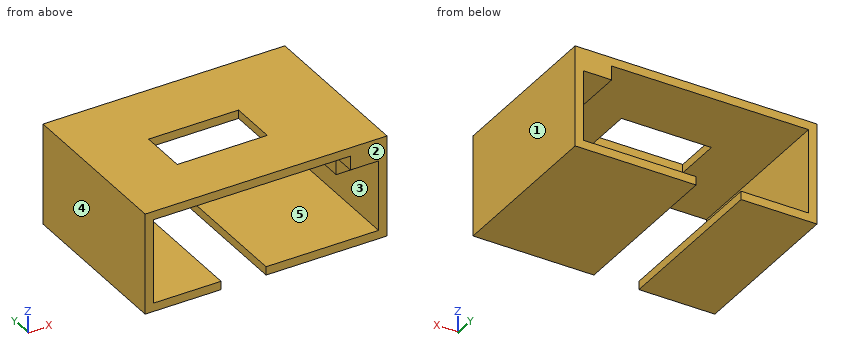
```python
from build123d import *

# Parameters (mm, degrees)
F1_DEPTH = 300
F2_W     = 160
F2_H     = 84.39811
F3_DEPTH = 25
F4_W     = 80
F4_H     = 50
F5_DEPTH = 30


with BuildPart() as f1:
    # F0 (on Front) → F1 (new body)
    with BuildSketch(Plane.XZ):
        Polygon((-80, -15), (-80, 0), (-200, 0), (-200, 150), (150, 150), (150, 125), (200, 125), (200, 0), (0, 0), (0, -15), (215, -15), (215, 165), (-215, 165), (-215, -15), align=None)
    extrude(amount=F1_DEPTH)

    # F2 (on face) → F3 (cut)
    with BuildSketch(Plane.XY.offset(165)):
        with Locations((-20, -162.199055)):
            Rectangle(F2_W, F2_H)
    extrude(amount=-F3_DEPTH, mode=Mode.SUBTRACT)

    # F4 (on face) → F5 (join)
    with BuildSketch(Plane(origin=(200, 0, 0), x_dir=(0, -1, 0), z_dir=(-1, 0, 0))):
        with Locations((185, 94.528437)):
            Rectangle(F4_W, F4_H)
    extrude(amount=F5_DEPTH)


solid = f1.part
```
Verification items for the finished model (mm, model axes). Face numbers are marked on the shaded views. A direction names the side the tool comes from. Round coordinates to 2 decimals unless told otherwise and drop trailing zeros. Order: outer loops, then holes, each group sorted by start corner. A loop starts at its lowest first (then second) coordinate and runs counter-clockwise, first axis right, second up. Notation, with made-up numbers: (41, 36) -> (53, 36) arc R24 cw to (53, 48) -> close; hole circle Ø10 at (12, 68.25). An arc over 180 degrees is marked (long way). Put each result on its own line as item: value. Start each with the question number.
(1) Tool access check on the marked faces 4 and 5. Record the directions out of +Z, -Z, +X, -X, +Y, -Y that give a thin tool (end or side, any length) a straight path to the whole face; none if there is none.
(2) Depth check by flat-ended pin: pin 1 Ø24 at (x, z) = (180.5, 97.5) entering from -Y; pin 2 Ø15 at (x, z) = (177.5, 95) entering from +Y; pin 3 Ø6 at (x, y) = (-42.5, -226) entering from -Z. Enter the tip coordinate at first touch or a pass-through.
(3) Material ranges on line 1 along X through (y, z) = (-51.5, 24); line 2 along Z through (x, y) = (196, -264); line 3 along Z through (x, y) = (-156.5, -111.5), recorded low to high.
(4) Section check A-A (x = -61). Enter the section's corners in (y, z), then the cut area to 3 significant figures.
(5) Draft check along X on the marked faces 1, 2 and 3. Enter one of: +X half, -X half, draft (parallel to the pull), parting line (faces both ways), or undercut.
(6) Section check C-C (y = -219). Enter the section's corners in (x, z).
(7) Section check D-D (x = 184). Enter the section's corners in (y, z).
(8) Section check B-B (z = 115). Enter the section's corners in (x, y).
Completed:
1. face 4: +Z, -Z, -X, +Y, -Y
1. face 5: +Y, -Y
2. pin 1: stops at y = -225
2. pin 2: stops at y = -145
2. pin 3: stops at z = 150
3. line 1: x = -215 to -200, 200 to 215
3. line 2: z = -15 to 0, 125 to 165
3. line 3: z = -15 to 0, 150 to 165
4. outline: (-300, 150) -> (-204.4, 150) -> (-204.4, 165) -> (-300, 165) -> close; (-120, 150) -> (0, 150) -> (0, 165) -> (-120, 165) -> close
4. area: 3,230 mm2
5. face 1: +X half
5. face 2: draft
5. face 3: undercut
6. outline: (-215, -15) -> (-80, -15) -> (-80, 0) -> (-200, 0) -> (-200, 150) -> (150, 150) -> (150, 125) -> (200, 125) -> (200, 119.53) -> (170, 119.53) -> (170, 69.53) -> (200, 69.53) -> (200, 0) -> (0, 0) -> (0, -15) -> (215, -15) -> (215, 165) -> (-215, 165) -> close
7. outline: (-300, -15) -> (0, -15) -> (0, 0) -> (-300, 0) -> close; (-300, 125) -> (0, 125) -> (0, 165) -> (-300, 165) -> close; (-225, 69.53) -> (-145, 69.53) -> (-145, 119.53) -> (-225, 119.53) -> close
8. outline: (-215, -300) -> (-200, -300) -> (-200, 0) -> (-215, 0) -> close; (170, -225) -> (200, -225) -> (200, -300) -> (215, -300) -> (215, 0) -> (200, 0) -> (200, -145) -> (170, -145) -> close
